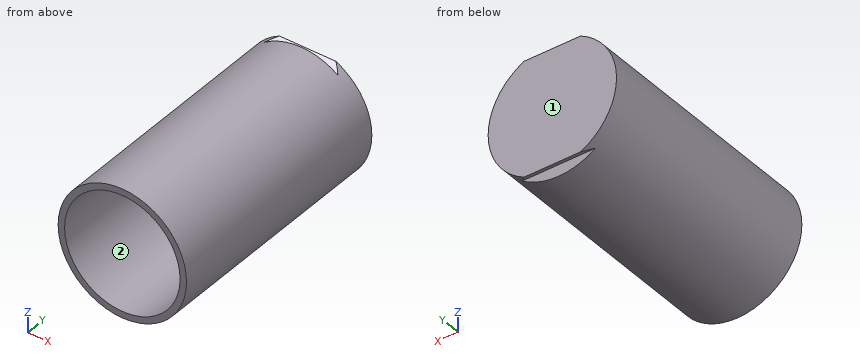
from build123d import *

# Parameters (mm, degrees)
F0_R      = 25
F1_DEPTH  = 90
F2_T      = -2.5
F1_FACE_R = 25
F3_DEPTH  = 6
F5_DEPTH  = 50


with BuildPart() as f1:
    # F0 (on Front) → F1 (new body)
    with BuildSketch(Plane.XZ):
        Circle(F0_R)
    extrude(amount=F1_DEPTH)

    # F2
    f2_openings = [f1.faces().sort_by_distance(p)[0] for p in [
        (0, -90, 0),
    ]]
    offset(amount=F2_T, openings=f2_openings)

    # F1_face (on face) → F3 (join)
    with BuildSketch(Plane(origin=(0, 0, 0), x_dir=(1, 0, 0), z_dir=(0, 1, 0))):
        Circle(F1_FACE_R)
    extrude(amount=F3_DEPTH)

    # F4 (on Right) → F5 (cut, symmetric)
    with BuildSketch(Plane.YZ):
        Polygon((2.675209, 35.80374), (2.675209, 20.530431), (6, 22.45), (6, 35.80374), align=None)
        Polygon((6, -37.240567), (6, -22.45), (2.675209, -20.530431), (2.675209, -37.240567), align=None)
    extrude(amount=F5_DEPTH, both=True, mode=Mode.SUBTRACT)


solid = f1.part
Can you work these out from the model? Positions are in its coordinate system, mm. Face numbers are marked on the shaded views. A direction names the side the tool comes from. Round coordinates to 2 decimals unless told otherwise and drop trailing zeros. Loops run counter-clockwise (first coordinate to the right, second up) from the corner with the lowest first, then second, coordinate; pieces in that order, holes last. Notation, with made-up numbers: (82, 64) - (104, 64) arc R17 ccw to (104, 80) - close; hole circle Ø3 at (17, 60.5). An arc over 180 degrees is marked (long way). Use CSV: the item, a comma, the result in double quotes. Start each with the question number.
1) If we section it at D-D on z = -13: Write out the boundary of the cut face in (x, y), plus the area to 3 significant figures.
2) Please list where these lines run through material, in increasing order: probe 1 along X at (y, z) = (-38, 0); probe 2 along Y at (x, z) = (14.5, 16). Write a range as [from, to].
3) For pin 1 Ø8 at (y, z) = (-64, 19.5) entering from +X; pin 2 Ø6 at (y, z) = (-35.5, 18) entering from +X; pin 3 Ø6 at (x, y) = (17, -22.5) entering from -Z, each with a flat end and sliding along its axis, tell me the tip position at first contact or that it passes through.
4) If we section it at B-B on z = 0: Write out the boundary of the cut face in (x, y), plus the area to 4 significant figures.
5) If we section it at A-A on x = 0: Write out the boundary of the cut face in (y, z).
6) For the marked faces 1 and 2, which set-ups out of +Z, -Z, +X, -X, +Y, -Y let a thin tool reach every point of the face, with its end or its side?
7) If we section it at C-C on y = -62: Write out the boundary of the cut face in (x, z).
Geometry results:
1,outline,"(-21.35, -90) - (-18.36, -90) - (-18.36, -2.5) - (18.36, -2.5) - (18.36, -90) - (21.35, -90) - (21.35, 6) - (-21.35, 6) - close"
1,area,"886 mm2"
2,probe 1,"x = [-25, -22.5], [22.5, 25]"
2,probe 2,"y = [-2.5, 6]"
3,pin 1,"stops at x = 19.62"
3,pin 2,"stops at x = 20"
3,pin 3,"stops at z = -20.71"
4,outline,"(-25, -90) - (-22.5, -90) - (-22.5, -2.5) - (22.5, -2.5) - (22.5, -90) - (25, -90) - (25, 6) - (-25, 6) - close"
4,area,"862.5 mm2"
5,outline,"(-90, -25) - (2.68, -25) - (2.68, -20.53) - (6, -22.45) - (6, 22.45) - (2.68, 20.53) - (2.68, 25) - (-90, 25) - (-90, 22.5) - (-2.5, 22.5) - (-2.5, -22.5) - (-90, -22.5) - close"
6,face 1,"+Z, -Z, +X, -X, +Y"
6,face 2,"-Y"
7,outline,"circle Ø50 at (0, 0); hole circle Ø45 at (0, 0)"
